Geometry check sheet. Reference: the model listing, model coordinates, mm. Face numbers are marked on the shaded views. Round coordinates to 2 decimals unless told otherwise and drop trailing zeros. Order: outer loops, then holes, each group sorted by start corner. A loop starts at its lowest first (then second) coordinate and runs counter-clockwise, first axis right, second up. Notation, with made-up numbers: (22, 62) - (45, 62) arc R28 ccw to (45, 90) - close; hole circle Ø3 at (-28, 36.5). An arc over 180 degrees is marked (long way). One line per question, with ' | ' between items. Start each with the question number.
Q1. Sectioned sample at C-C, the plane y = 19. Give the number of separate pieces and of enclosed holes in the cut face, then the cut area to 3 significant figures.
Q2. Sectioned sample at A-A, the plane z = 0. Enter the section's corners in (x, y) (3 decimals), then the cut area to 3 significant figures.
Q3. Sectioned sample at B-B, the plane x = -42. Enter the section's corners in (y, z) (3 decimals).
Q4. Mould release check, pull along X, two halves, no side actions. Record for the marked faces 1, 2 and 3: +X half, -X half, draft (parallel to the pull), parting line (faces both ways), or undercut.
Q5. Sectioned sample at D-D, the plane z = 28. Enter the section's corners in (x, y), then the cut area to 3 significant figures.
Q6. Material ranges on line 1 along X through (y, z) = (47.5, -2.5); line 2 along X through (y, z) = (8, -21.5); line 3 along Z through (x, y) = (-31.5, 24.5) (3 decimals), recorded low to high.
Q7. Gauge pin test, flat ends, axial feed: P1, Ø8, axis at x = -42.5, y = 25.5, coming from the -Z side; P2, Ø1.2, axis at y = 37.5, z = -30.5, coming from the +X side (3 decimals); P3, Ø1.2, axis at x = -52, y = 35, coming from the -Z side. Record the tip position at first contact, or that the pin passes through.
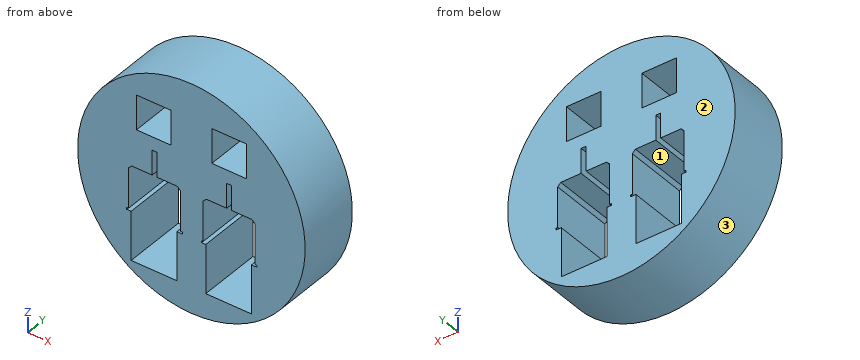
```python
from build123d import *

# Parameters (mm, degrees)
SKETCH1_R           = 92.075
BOSS_EXTRUDE1_DEPTH = 50.8
SKETCH6_W           = 27.94
SKETCH6_H           = 27.94
CUT_EXTRUDE4_DEPTH  = 50.8
CUT_EXTRUDE5_DEPTH  = 50.8


with BuildPart() as part:
    # Sketch1 → Boss-Extrude1 (new body)
    with BuildSketch(Plane(origin=(0, 0, 0), x_dir=(1, 0, 0), z_dir=(0, 1, 0))):
        with Locations(Location((0, 0, 0), (0, 0, 270))):
            Circle(SKETCH1_R)
    extrude(amount=BOSS_EXTRUDE1_DEPTH)

    # Sketch6 → Cut-Extrude4 (cut)
    with BuildSketch(Plane.XZ):
        with Locations((30.48, 49.53)):
            Rectangle(SKETCH6_W, SKETCH6_H)
        with Locations((-30.48, 49.53)):
            Rectangle(SKETCH6_W, SKETCH6_H)
    extrude(amount=-CUT_EXTRUDE4_DEPTH, mode=Mode.SUBTRACT)

    # Sketch8 → Cut-Extrude5 (cut)
    with BuildSketch(Plane(origin=(0, 50.8, 0), x_dir=(1, 0, 0), z_dir=(0, 1, 0))):
        Polygon((48.673227998, 66.920620093), (48.673227998, 31.675), (53.066023648, 31.675), (53.066023648, 30.175), (51.568299971, 30.175), (51.568299971, -2.285), (49.028299971, -4.825), (32.568299971, -4.825), (32.568299971, -24.825), (28.568299971, -24.825), (28.568299971, -4.825), (12.108299971, -4.825), (9.568299971, -2.285), (9.568299971, 30.175), (8.06602381, 30.175), (8.06602381, 31.675), (10.838299971, 31.675), (11.658892904, 31.675), (11.658892904, 66.920620093), (11.658892904, 71.12), (48.673227998, 71.12), align=None)
        Polygon((-8.831700029, -2.285), (-11.371700029, -4.825), (-27.831700029, -4.825), (-27.831700029, -24.825), (-31.831700029, -24.825), (-31.831700029, -4.825), (-48.291700029, -4.825), (-50.831700029, -2.285), (-50.831700029, 30.175), (-52.33397619, 30.175), (-52.33397619, 31.675), (-48.741107096, 31.675), (-48.741107096, 66.920620093), (-48.741107096, 71.12), (-11.726772002, 71.12), (-11.726772002, 66.920620093), (-11.726772002, 31.675), (-7.333976352, 31.675), (-7.333976352, 30.175), (-8.831700029, 30.175), align=None)
    extrude(amount=-CUT_EXTRUDE5_DEPTH, mode=Mode.SUBTRACT)


solid = part.part
```
Determined:
1) separate pieces: 1 | enclosed holes: 4 | area: 18,900 mm2
2) outline: (-92.075, 0) - (-50.832, 0) - (-50.832, 50.8) - (-92.075, 50.8) - close; (-8.832, 0) - (9.568, 0) - (9.568, 50.8) - (-8.832, 50.8) - close; (51.568, 0) - (92.075, 0) - (92.075, 50.8) - (51.568, 50.8) - close | area: 5,090 mm2
3) outline: (0, -81.938) - (50.8, -81.938) - (50.8, -71.12) - (0, -71.12) - close; (0, 4.825) - (50.8, 4.825) - (50.8, 35.56) - (0, 35.56) - close; (0, 63.5) - (50.8, 63.5) - (50.8, 81.938) - (0, 81.938) - close
4) face 1: undercut | face 2: draft | face 3: parting line
5) outline: (-87.71, 0) - (87.71, 0) - (87.71, 50.8) - (-87.71, 50.8) - close | area: 8,910 mm2
6) line 1: x = -92.04 to -50.83, -8.83 to 9.57, 51.57 to 92.04 | line 2: x = -89.53 to -50.83, -8.83 to 9.57, 51.57 to 89.53 | line 3: z = -86.519 to -71.12, 24.825 to 35.56, 63.5 to 86.519
7) P1: stops at z = -83.64 | P2: stops at x = 87.085 | P3: stops at z = -76.39
